from build123d import *

# Parameters (mm, degrees)
CHAMFER1_SIZE = 0.5
FILLET1_R     = 1
CHAMFER2_SIZE = 0.5


with BuildPart() as part:
    # Sketch1 → Revolve1 (revolve)
    with BuildSketch(Plane.XY):
        Polygon((1.493038446, 27.8), (11, 33.23), (11, 49.2), (17.45, 49.2), (17.45, 6.25), (25, 6.25), (25, 3), (21.75, 3), (21.75, 0), (12.334639896, 0), (12.334639896, 25.3), (1.493038446, 25.3), align=None)
    revolve(axis=Axis((0, 0, 0), (0, 1, 0)))

    # Chamfer1
    chamfer1_edges = [part.edges().sort_by_distance(p)[0] for p in [
        (-11, 49.2, 0),
        (-17.45, 49.2, 0),
        (-25, 6.25, 0),
        (-25, 3, 0),
        (-21.75, 0, 0),
        (-12.334639896, 0, 0),
        (-1.493038446, 25.3, 0),
    ]]
    chamfer(chamfer1_edges, length=CHAMFER1_SIZE)

    # Fillet1
    fillet1_edges = [part.edges().sort_by_distance(p)[0] for p in [
        (-17.45, 6.25, 0),
    ]]
    fillet(fillet1_edges, radius=FILLET1_R)

    # Chamfer2
    chamfer2_edges = [part.edges().sort_by_distance(p)[0] for p in [
        (-12.334639896, 25.3, 0),
    ]]
    chamfer(chamfer2_edges, length=CHAMFER2_SIZE)


solid = part.part
The listing builds one solid part. Answer for the finished solid, in the listing's coordinates (mm). A direction names the side the tool comes from. Give positions to 0.01 mm unless a question says otherwise; leave off trailing zeros. Write each loop counter-clockwise with the first axis right and the second up, starting at its lowest first coordinate (ties: lowest second). Pieces come first, ordered by that corner, then holes.
1) Section A-A (y = 5) is taken. Write down the section's boundary in (x, z).
2) Section B-B (y = 15.5) is taken. Write down the section's boundary in (x, z).
3) Given P1, Ø13, axis at x = 0, z = 0, coming from the -Y side; P2, Ø4, axis at y = 16.5, z = -6.5, coming from the -X side; P3, Ø1, axis at x = 3.5, y = 8.5, coming from the +Z side, each flat-ended and moving along its own axis, determine where each tip first touches the part or whether it passes through.
4) For a pull along Z with two mould halves and no side action, classify faces 4 (the face through (-11, 49.2, 4)), 5 (the face through (-0.19, 26.81, -1.48)), 6 (the face through (-3.783, 27.685, 17.035)) as pulls with the +Z half, pulls with the -Z half, needs draft (parallel to the pull), parting line crosses it, or undercut.
5) Find the intervals of material crossed by L1, parallel to Z at x = 0, y = 12.25; L2, parallel to Z at x = 0, y = 43.5, in increasing order.
6) A tool of negligible diameter and unlimited length cuts with its end or side. For faces 1 (the face through (-3.5, 6.25, -18.3)), 2 (the face through (23.846, 4.609, -7.509)), 3 (the face through (0, 3, -22)), from which of +Z, -Z, +X, -X, +Y, -Y can it reach the whole face along a straight path? Write none if from no direction.
Response:
1. outline: circle Ø50 at (0, 0); hole circle Ø24.67 at (0, 0)
2. outline: circle Ø34.9 at (0, 0); hole circle Ø24.67 at (0, 0)
3. P1: stops at y = 25.3
3. P2: stops at x = -16.86
3. P3: stops at z = 17.19
4. face 4: needs draft
4. face 5: undercut
4. face 6: parting line crosses it
5. L1: z = -17.45 to -12.33, 12.33 to 17.45
5. L2: z = -17.45 to -11, 11 to 17.45
6. face 1: +Y
6. face 2: +Y, -Y
6. face 3: -Y
